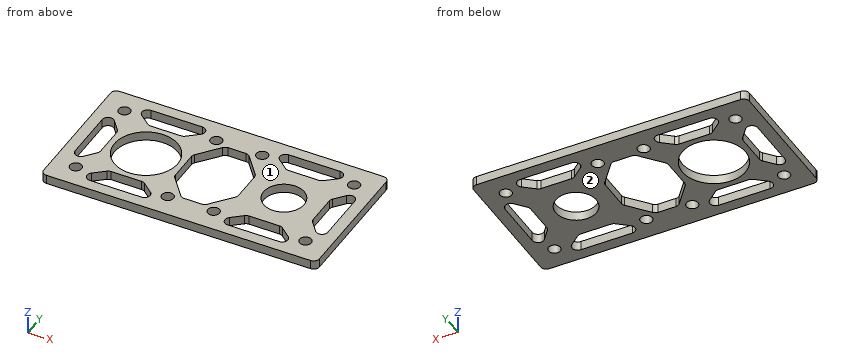
from build123d import *

# Parameters (mm, degrees)
SKETCH1_W           = 96
SKETCH1_H           = 48
SKETCH1_R           = 2.05
SKETCH1_R_2         = 11
SKETCH1_R_3         = 7.05
BOSS_EXTRUDE1_DEPTH = 3.175
FILLET1_R           = 2


with BuildPart() as part:
    # Sketch1 → Boss-Extrude1 (new body)
    with BuildSketch(Plane.XY):
        Rectangle(SKETCH1_W, SKETCH1_H)
        with Locations((-40, 16)):
            Circle(SKETCH1_R, mode=Mode.SUBTRACT)
        with Locations((-8, 16)):
            Circle(SKETCH1_R, mode=Mode.SUBTRACT)
        with Locations((-8, -16)):
            Circle(SKETCH1_R, mode=Mode.SUBTRACT)
        with Locations((-40, -16)):
            Circle(SKETCH1_R, mode=Mode.SUBTRACT)
        with Locations((-24, 0)):
            Circle(SKETCH1_R_2, mode=Mode.SUBTRACT)
        with Locations(Location((8, 16, 0), (0, 0, 180))):
            Circle(SKETCH1_R, mode=Mode.SUBTRACT)
        with Locations(Location((8, -16, 0), (0, 0, 180))):
            Circle(SKETCH1_R, mode=Mode.SUBTRACT)
        with Locations(Location((40, -16, 0), (0, 0, 180))):
            Circle(SKETCH1_R, mode=Mode.SUBTRACT)
        with Locations(Location((40, 16, 0), (0, 0, 180))):
            Circle(SKETCH1_R, mode=Mode.SUBTRACT)
        with Locations((24, 0)):
            Circle(SKETCH1_R_3, mode=Mode.SUBTRACT)
        Polygon((-38.544929421, 20.05), (-30, 13), (-18, 13), (-9.455070579, 20.05), align=None, mode=Mode.SUBTRACT)
        Polygon((-18, -13), (-9.455070579, -20.05), (-38.544929421, -20.05), (-30, -13), align=None, mode=Mode.SUBTRACT)
        Polygon((-11, -6), (-11, 6), (-4, 14.484327085), (4, 14.484327085), (11, 6), (11, -6), (4, -14.484327085), (-4, -14.484327085), align=None, mode=Mode.SUBTRACT)
        Polygon((30, -13), (18, -13), (9.455070579, -20.05), (38.544929421, -20.05), align=None, mode=Mode.SUBTRACT)
        Polygon((37, -6), (37, 6), (44, 14.484327085), (44, -14.484327085), align=None, mode=Mode.SUBTRACT)
        Polygon((18, 13), (9.455070579, 20.05), (38.544929421, 20.05), (30, 13), align=None, mode=Mode.SUBTRACT)
        Polygon((-44, -14.484327085), (-37, -6), (-37, 6), (-44, 14.484327085), align=None, mode=Mode.SUBTRACT)
    extrude(amount=BOSS_EXTRUDE1_DEPTH)

    # Fillet1
    fillet1_edges = [part.edges().sort_by_distance(p)[0] for p in [
        (38.544929421, -20.05, 1.5875),
        (30, -13, 1.5875),
        (18, -13, 1.5875),
        (9.455070579, -20.05, 1.5875),
        (37, -6, 1.5875),
        (44, -14.484327085, 1.5875),
        (44, 14.484327085, 1.5875),
        (37, 6, 1.5875),
        (18, 13, 1.5875),
        (30, 13, 1.5875),
        (38.544929421, 20.05, 1.5875),
        (9.455070579, 20.05, 1.5875),
        (-9.455070579, 20.05, 1.5875),
        (-38.544929421, 20.05, 1.5875),
        (-30, 13, 1.5875),
        (-18, 13, 1.5875),
        (-11, -6, 1.5875),
        (-4, -14.484327085, 1.5875),
        (4, -14.484327085, 1.5875),
        (11, -6, 1.5875),
        (11, 6, 1.5875),
        (4, 14.484327085, 1.5875),
        (-4, 14.484327085, 1.5875),
        (-11, 6, 1.5875),
        (-37, -6, 1.5875),
        (-37, 6, 1.5875),
        (-44, 14.484327085, 1.5875),
        (-44, -14.484327085, 1.5875),
        (-48, 24, 1.5875),
        (48, 24, 1.5875),
        (48, -24, 1.5875),
        (-48, -24, 1.5875),
        (-18, -13, 1.5875),
        (-30, -13, 1.5875),
        (-38.544929421, -20.05, 1.5875),
        (-9.455070579, -20.05, 1.5875),
    ]]
    fillet(fillet1_edges, radius=FILLET1_R)


solid = part.part
Build history of the part. All positions in model axes, mm. Face numbers are marked on the shaded views. Round coordinates to 2 decimals unless told otherwise and drop trailing zeros. Loops run counter-clockwise (first coordinate to the right, second up) from the corner with the lowest first, then second, coordinate; pieces in that order, holes last. Notation, with made-up numbers: (-1.75, 16.5) -> (22.25, 16.5) arc R17 ccw to (22.25, 37.5) -> close; hole circle Ø5 at (-34.75, 24.5). An arc over 180 degrees is marked (long way). One line per item, written item: value. Start each with the question number.
Q1. Probe line 1 along Y through (x, z) = (24, 1.9); line 2 along Y through (x, z) = (-23.5, 0.2); line 3 along X through (y, z) = (0.5, 2.7). List the from-to ranges inside material, lowest first.
Q2. Cut at D-D on y = 8. List the corners of the cut face in (x, z) (3 decimals).
Q3. Cut at A-A on x = -24. List the corners of the cut face in (y, z) (3 decimals).
Q4. Cut at C-C on z = 2. Count the separate pieces of the cut face and the enclosed holes in it, plus the area to 3 significant figures.
Q5. Drop flat-ended pins along their axis: pin 1 Ø17.5 at (x, y) = (-24, 0) entering from +Z; pin 2 Ø6.5 at (x, y) = (8, -16) entering from +Z (3 decimals). Give the stop position or say it passes through.
Q6. Two-plate mould, pull along Z, no slides. Class the marked faces 1 and 2: released by +Z, released by -Z, zero draft, split by the parting line, or undercut.
Q7. Cut at B-B on y = 0. List the corners of the cut face in (x, z) (3 decimals), plus the area to 3 significant figures.
Computed:
1. line 1: -24 to -20.05, -13 to -7.05, 7.05 to 13, 20.05 to 24
1. line 2: -24 to -20.05, -13 to -10.99, 10.99 to 13, 20.05 to 24
1. line 3: -48 to -44, -37 to -34.99, -13.01 to -11, 11 to 16.97, 31.03 to 37, 44 to 48
2. outline: (-48, 0) -> (-44, 0) -> (-44, 3.175) -> (-48, 3.175) -> close; (-38.65, 0) -> (-31.55, 0) -> (-31.55, 3.175) -> (-38.65, 3.175) -> close; (-16.45, 0) -> (-9.35, 0) -> (-9.35, 3.175) -> (-16.45, 3.175) -> close; (9.35, 0) -> (38.65, 0) -> (38.65, 3.175) -> (9.35, 3.175) -> close; (44, 0) -> (48, 0) -> (48, 3.175) -> (44, 3.175) -> close
3. outline: (-24, 0) -> (-20.05, 0) -> (-20.05, 3.175) -> (-24, 3.175) -> close; (-13, 0) -> (-11, 0) -> (-11, 3.175) -> (-13, 3.175) -> close; (11, 0) -> (13, 0) -> (13, 3.175) -> (11, 3.175) -> close; (20.05, 0) -> (24, 0) -> (24, 3.175) -> (20.05, 3.175) -> close
4. separate pieces: 1
4. enclosed holes: 17
4. area: 2,650 mm²
5. pin 1: through
5. pin 2: z = 3.175
6. face 1: released by +Z
6. face 2: released by -Z
7. outline: (-48, 0) -> (-44, 0) -> (-44, 3.175) -> (-48, 3.175) -> close; (-37, 0) -> (-35, 0) -> (-35, 3.175) -> (-37, 3.175) -> close; (-13, 0) -> (-11, 0) -> (-11, 3.175) -> (-13, 3.175) -> close; (11, 0) -> (16.95, 0) -> (16.95, 3.175) -> (11, 3.175) -> close; (31.05, 0) -> (37, 0) -> (37, 3.175) -> (31.05, 3.175) -> close; (44, 0) -> (48, 0) -> (48, 3.175) -> (44, 3.175) -> close
7. area: 75.9 mm²
